The listing builds one solid part. Answer for the finished solid, in the listing's coordinates (mm). A direction names the side the tool comes from. Round coordinates to 2 decimals unless told otherwise and drop trailing zeros. Write each loop counter-clockwise with the first axis right and the second up, starting at its lowest first coordinate (ties: lowest second). Pieces come first, ordered by that corner, then holes.
from build123d import *

# Parameters (mm, degrees)
SKETCH_R        = 3.1
SKETCH_R_2      = 4
SKETCH_R_3      = 2
SKETCH_R_4      = 2.1
PAD_DEPTH       = 8
SKETCH001_R     = 11.1
POCKET_DEPTH    = 3
SKETCH002_R     = 5
SKETCH002_R_2   = 6
POCKET001_DEPTH = 2
SKETCH003_R     = 11.1
POCKET002_DEPTH = 3
FILLET_R        = 4
FILLET001_R     = 4
FILLET002_R     = 4
FILLET003_R     = 4
FILLET004_R     = 4


with BuildPart() as part:
    # Sketch → Pad (new body)
    with BuildSketch(Plane.XY):
        Polygon((0, 0), (0, 56), (60, 56), (60, 40), (100, 40), (100, 0), align=None)
        with Locations((90, 30)):
            Circle(SKETCH_R, mode=Mode.SUBTRACT)
        with Locations((70, 30)):
            Circle(SKETCH_R, mode=Mode.SUBTRACT)
        with Locations((38.85, 30)):
            Circle(SKETCH_R_2, mode=Mode.SUBTRACT)
        with Locations((23.35, 45.5)):
            Circle(SKETCH_R_3, mode=Mode.SUBTRACT)
        with Locations((23.35, 14.5)):
            Circle(SKETCH_R_3, mode=Mode.SUBTRACT)
        with Locations((54.35, 14.5)):
            Circle(SKETCH_R_3, mode=Mode.SUBTRACT)
        with Locations((54.35, 45.5)):
            Circle(SKETCH_R_3, mode=Mode.SUBTRACT)
        with Locations((6, 6)):
            Circle(SKETCH_R_4, mode=Mode.SUBTRACT)
        with Locations((6, 50)):
            Circle(SKETCH_R_4, mode=Mode.SUBTRACT)
        with Locations((90, 6)):
            Circle(SKETCH_R_4, mode=Mode.SUBTRACT)
        with Locations((70, 6)):
            Circle(SKETCH_R_4, mode=Mode.SUBTRACT)
    extrude(amount=PAD_DEPTH)

    # Sketch001 → Pocket (cut)
    with BuildSketch(Plane.XY.offset(8)):
        with Locations((38.85, 30)):
            Circle(SKETCH001_R)
    extrude(amount=-POCKET_DEPTH, mode=Mode.SUBTRACT)

    # Sketch002 → Pocket001 (cut)
    with BuildSketch(Plane.XY.offset(8)):
        with Locations((6, 50)):
            Circle(SKETCH002_R)
        with Locations((6, 6)):
            Circle(SKETCH002_R)
        with Locations((70, 6)):
            Circle(SKETCH002_R)
        with Locations((90, 6)):
            Circle(SKETCH002_R)
        with Locations((70, 30)):
            Circle(SKETCH002_R_2)
        with Locations((90, 30)):
            Circle(SKETCH002_R_2)
    extrude(amount=-POCKET001_DEPTH, mode=Mode.SUBTRACT)

    # Sketch003 → Pocket002 (cut)
    with BuildSketch(Plane(origin=(0, 0, 0), x_dir=(1, 0, 0), z_dir=(0, 0, -1))):
        with Locations((38.85, -30)):
            Circle(SKETCH003_R)
    extrude(amount=-POCKET002_DEPTH, mode=Mode.SUBTRACT)

    # Fillet
    fillet_edges = [part.edges().sort_by_distance(p)[0] for p in [
        (0, 56, 4),
    ]]
    fillet(fillet_edges, radius=FILLET_R)

    # Fillet001
    fillet001_edges = [part.edges().sort_by_distance(p)[0] for p in [
        (60, 56, 4),
    ]]
    fillet(fillet001_edges, radius=FILLET001_R)

    # Fillet002
    fillet002_edges = [part.edges().sort_by_distance(p)[0] for p in [
        (100, 40, 4),
    ]]
    fillet(fillet002_edges, radius=FILLET002_R)

    # Fillet003
    fillet003_edges = [part.edges().sort_by_distance(p)[0] for p in [
        (100, 0, 4),
    ]]
    fillet(fillet003_edges, radius=FILLET003_R)

    # Fillet004
    fillet004_edges = [part.edges().sort_by_distance(p)[0] for p in [
        (0, 0, 4),
    ]]
    fillet(fillet004_edges, radius=FILLET004_R)


solid = part.part
1. Section C-C on y = 6 is taken. Determine the outline of the cut face in (x, z), plus the area to 3 significant figures.
Geometry says:
outline: (0, 0) - (3.9, 0) - (3.9, 6) - (1, 6) - (1, 8) - (0, 8) - close; (8.1, 0) - (67.9, 0) - (67.9, 6) - (65, 6) - (65, 8) - (11, 8) - (11, 6) - (8.1, 6) - close; (72.1, 0) - (87.9, 0) - (87.9, 6) - (85, 6) - (85, 8) - (75, 8) - (75, 6) - (72.1, 6) - close; (92.1, 0) - (100, 0) - (100, 8) - (95, 8) - (95, 6) - (92.1, 6) - close
area: 664 mm2
2. Straight lines are drawn through the part: line 1 along Y through (x, z) = (54.35, 4); line 2 along Y through (x, z) = (90, 2.6); line 3 along X through (y, z) = (45, 1). For each, find the intervals that lie inside material, in ascending order.
Geometry says:
line 1: y = 0 to 12.5, 16.5 to 43.5, 47.5 to 56
line 2: y = 0 to 3.9, 8.1 to 26.9, 33.1 to 40
line 3: x = 0 to 21.41, 25.29 to 52.41, 56.29 to 60
3. Section B-B on z = 1 is taken. Give the number of separate pieces and of enclosed holes in the cut face, plus the area to 3 significant figures.
Geometry says:
separate pieces: 1
enclosed holes: 11
area: 4,390 mm2
4. Given pin 1 (2 mm diameter, centred on y = 38.5, z = 2, fed in from +X); pin 2 (2.5 mm diameter, centred on x = 77.5, z = 4.5, fed in from +Y); pin 3 (4 mm diameter, centred on y = 46, z = 3, fed in from +X), each flat-ended and moving along its own axis, determine where each tip first touches the part or whether it passes through.
Geometry says:
pin 1: stops at x = 99.71
pin 2: stops at y = 40
pin 3: stops at x = 60
5. For a pull along Y with two mould halves and no side action, classify faces 1 (the face through (51, 22, 0)), 2 (the face through (51, 0, 4)), 3 (the face through (74.619, 4.085, 7.014)), 4 (the face through (58.797, 54.859, 4.056)) as released by +Y, released by -Y, zero draft, split by the parting line, or undercut.
Geometry says:
face 1: zero draft
face 2: released by -Y
face 3: undercut
face 4: released by +Y
6. Section A-A on x = 38.85 is taken. Determine the outline of the cut face in (y, z).
Geometry says:
outline: (0, 0) - (18.9, 0) - (18.9, 3) - (26, 3) - (26, 5) - (18.9, 5) - (18.9, 8) - (0, 8) - close; (34, 3) - (41.1, 3) - (41.1, 0) - (56, 0) - (56, 8) - (41.1, 8) - (41.1, 5) - (34, 5) - close
7. A tool of negligible diameter and unlimited length cuts with its end or side. For faces 5 (the face through (49.44, 33.33, 6.52)), 6 (the face through (44, 30, 3)), 7 (the face through (60, 46, 4)), from which of +Z, -Z, +X, -X, +Y, -Y can it reach the whole face along a straight path? Write none if from no direction.
Geometry says:
face 5: +Z
face 6: -Z
face 7: +Z, -Z, +X, +Y
8. Section D-D on x = 23.35 is taken. Determine the outline of the cut face in (y, z).
Geometry says:
outline: (0, 0) - (12.5, 0) - (12.5, 8) - (0, 8) - close; (16.5, 0) - (43.5, 0) - (43.5, 8) - (16.5, 8) - close; (47.5, 0) - (56, 0) - (56, 8) - (47.5, 8) - close
